```python
from build123d import *

# Parameters (mm, degrees)
F2_R     = 3.175
F3_DEPTH = 101.6


# Not quite as in the source:
# - a fillet or chamfer that OpenCascade refuses, or shapes differently, is made with other operations: its cross-section is extruded or revolved along the edge and cut away or added


with BuildPart() as f1:
    # F0 (on Front) → F1 (revolve)
    with BuildSketch(Plane.XZ):
        with BuildLine():
            ThreePointArc((0, -50.8), (50.8, 0), (0, 50.8))
            Line((0, 50.8), (0, 44.45))
            ThreePointArc((0, 44.45), (44.45, 0), (0, -44.45))
            Line((0, -44.45), (0, -50.8))
        make_face()
    revolve(axis=Axis((0, 0, 0), (0, 0, -1)))

    # F2 (on Front) → F3 (cut)
    with BuildSketch(Plane.XZ):
        Circle(F2_R)
    extrude(amount=-F3_DEPTH, mode=Mode.SUBTRACT)

    # F4: chamfer of 6.35 on 1 edges, made by hand

    # F4_s1 → F4_t2 (revolve, cut)
    with BuildSketch(Plane.XY.offset(-1.2e-09)):
        with BuildLine():
            Line((3.0138514094, 50.4834593112), (8.8272948956, 43.4006886388))
            Line((8.8272948956, 43.4006886388), (8.8025344773, 43.2761257162))
            ThreePointArc((8.8025344773, 43.2761257162), (6.0073622852, 43.914006044), (3.1659285713, 44.2097865329))
            Line((3.1659285713, 44.2097865329), (3.048, 44.336462139))
            ThreePointArc((3.048, 44.336462139), (3.047999955, 47.4099607251), (2.8868514094, 50.4834593112))
            Line((2.8868514094, 50.4834593112), (3.0138514094, 50.4834593112))
        make_face()
    revolve(axis=Axis((-2.25e-08, 44.336462139, -1.2e-09), (0, -1, 0)), mode=Mode.SUBTRACT)


solid = f1.part
```
The model under review builds one solid part; all positions refer to its coordinate system, in mm. A direction names the side the tool comes from. Coordinates: 2 decimals unless noted, no trailing zeros. Write each loop counter-clockwise with the first axis right and the second up, starting at its lowest first coordinate (ties: lowest second). Pieces come first, ordered by that corner, then holes.
1) To check wall thickness, follow probe 1 along Z at (x, y) = (6.5, -34.5); probe 2 along Z at (x, y) = (14, 15.5); probe 3 along X at (y, z) = (-4, -28.5). State the ranges of each line that lie inside material, in increasing order.
2) We need section B-B on x = 0. State the section outline as (y, z) points (3 decimals).
3) We need section C-C on z = 40. State the section outline as (x, y) points, then the cut area to 3 significant figures.
4) Machinability: for faces 1 (the face through (3.356, 49.869, 1.057)), 2 (the face through (-0.69, 50.49, -3.1)), which of the approach directions +Z, -Z, +X, -X, +Y, -Y give a long, thin tool a straight path to every point of the face, cutting with its end or side? Answer none if there is none.
5) We need section A-A on z = 0. State the section outline as (x, y) points (3 decimals).
6) Clearance check with flat-ended pins moving along their axes: pin 1 Ø1 at (y, z) = (25, 2) entering from +X; pin 2 Ø6 at (x, y) = (-5.5, -22.5) entering from +Z; pin 3 Ø6 at (y, z) = (36.5, 6.5) entering from +X. State where each tip first meets the part, or that it passes through.
7) We need section D-D on y = 26.5. State the section outline as (x, z) points.
Answer list:
1. probe 1: z = -36.72 to -27.26, 27.26 to 36.72
1. probe 2: z = -46.31 to -39.24, 39.24 to 46.31
1. probe 3: x = -41.86 to -33.88, 33.88 to 41.86
2. outline: (43.597, -8.666) arc R44.45 cw (long way) to (43.597, 8.666) - (50.287, 3.175) - (50.701, 3.175) arc R50.8 ccw (long way) to (50.701, -3.175) - (50.287, -3.175) - close
3. outline: circle Ø62.63 at (0, 0); hole circle Ø38.77 at (0, 0)
3. area: 1,900 mm2
4. face 1: none
4. face 2: +Y
5. outline: (-8.666, 43.597) - (-3.175, 50.287) - (-3.175, 50.701) arc R50.8 ccw (long way) to (3.175, 50.701) - (3.175, 50.287) - (8.666, 43.597) arc R44.45 cw (long way) to start
6. pin 1: stops at x = 44.46
6. pin 2: stops at z = 46.63
6. pin 3: stops at x = 37.68
7. outline: circle Ø86.68 at (0, 0); hole circle Ø71.37 at (0, 0)
